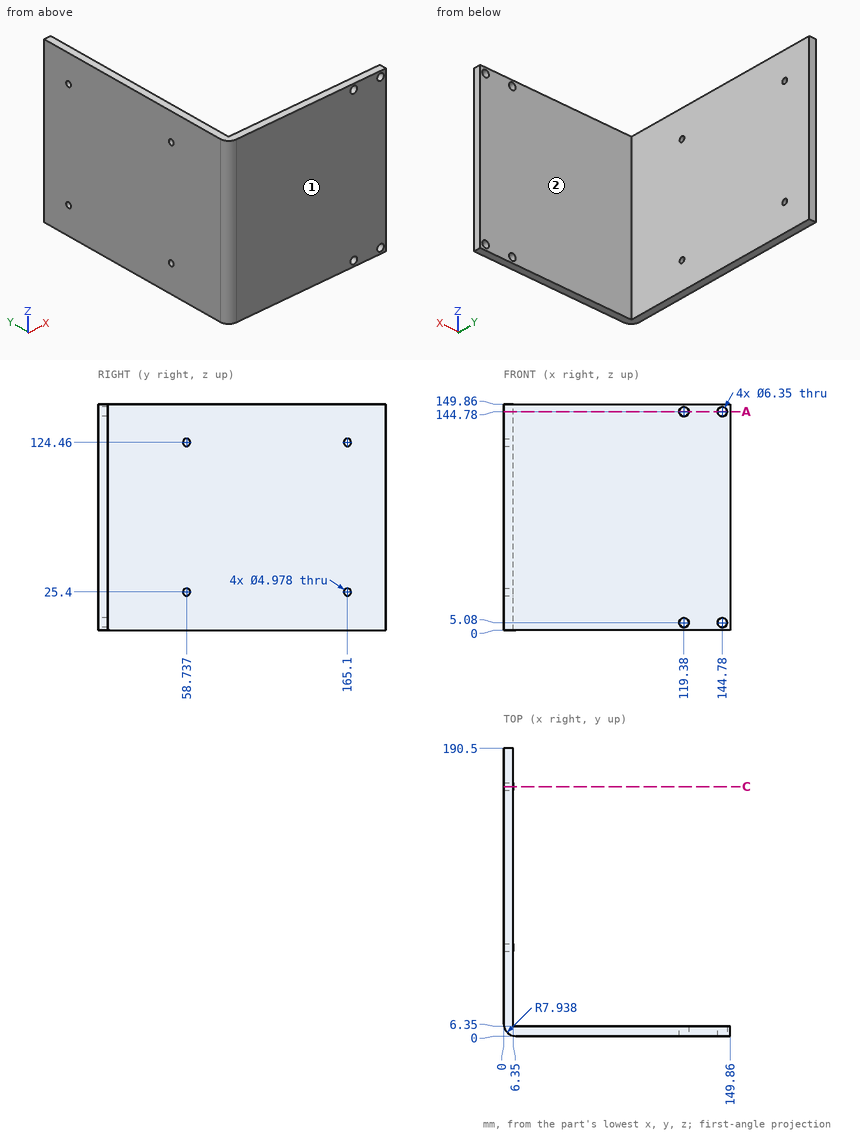
Verification items for this drawing (mm, ordinates from the low corner). A direction names the side the tool comes from. Coordinates: 2 decimals unless noted, no trailing zeros. Write each loop counter-clockwise with the first axis right and the second up, starting at its lowest first coordinate (ties: lowest second). Pieces come first, ordered by that corner, then holes. Notation, with made-up numbers: M 51.5,-14 L 56.5,-14 A23 cw 56.5,20 Z; hole C -31,79.25 d11. An arc over 180 degrees is marked long. Answer as a JSON object with one key per item and string values. Group by question number.
(1) Material ranges on line 1 (X direction, y = 2, z = 5) (1 decimal); line 2 (Z direction, x = 144, y = 2); line 3 (X direction, y = 121, z = 53), recorded low to high.
(2) Gauge pin test, flat ends, axial feed: pin 1 (4.5 mm diameter, centred on y = 58.74, z = 124.46, fed in from -X); pin 2 (10 mm diameter, centred on x = 122, z = 41.5, fed in from -Y); pin 3 (3 mm diameter, centred on x = 96, z = 65.5, fed in from +Y); pin 4 (2 mm diameter, centred on y = 57.5, z = 68.5, fed in from +X). Record the tip position at first contact, or that the pin passes through.
(3) Cross-section at A-A, the plane z = 144.78. State how many separate pieces and enclosed holes the cut face has, and give its area (3 significant figures).
(4) Cross-section at C-C, the plane y = 165.1. Record the cut outline in (x, z).
(5) Tool access check on the marked faces 1 and 2. Record the directions out of +Z, -Z, +X, -X, +Y, -Y that give a thin tool (end or side, any length) a straight path to the whole face; none if there is none.
Reply:
{
 "1": {"line 1": "2.7 to 116.2, 122.6 to 141.6, 148 to 149.9", "line 2": "0 to 2, 8.16 to 141.7, 147.86 to 149.86", "line 3": "0 to 6.35"},
 "2": {"pin 1": "through", "pin 2": "y = 0", "pin 3": "y = 6.35", "pin 4": "x = 6.35"},
 "3": {"separate pieces": "3", "enclosed holes": "0", "area": "2,030 mm²"},
 "4": {"outline": "M 0,0 L 6.35,0 L 6.35,22.91 L 0,22.91 Z; M 0,27.89 L 6.35,27.89 L 6.35,121.97 L 0,121.97 Z; M 0,126.95 L 6.35,126.95 L 6.35,149.86 L 0,149.86 Z"},
 "5": {"face 1": "+Z, -Z, +X, -X, -Y", "face 2": "+Z, -Z, +X, +Y"}
}
